```python
from build123d import *

# Parameters (mm, degrees)
SKETCH2_W                  = 60
SKETCH2_H                  = 60
BOSS_EXTRUDE1_DEPTH        = 7.5
BOSS_EXTRUDE2_DEPTH        = 15
FILLET1_R                  = 1
SKETCH4_R                  = 2.5
CUT_EXTRUDE1_DEPTH         = 57.024687639
CUT_EXTRUDE2_START         = -7.5
SKETCH5_R                  = 4.25
CUT_EXTRUDE2_DEPTH         = 7.5
CHAMFER3_SIZE              = 1
LPATTERN1_COUNT            = 5
LPATTERN1_PITCH            = 10
CHAMFER3_OF_LPATTERN1_SIZE = 1
CHAMFER1_SIZE              = 3
CHAMFER2_SIZE              = 1


# Read off the part's stored shape, not the designer's step: LPattern2
with BuildPart() as part:
    # Sketch2 → Boss-Extrude1 (new, symmetric)
    with BuildSketch(Plane(origin=(0, 0, 0), x_dir=(0, 1, 0), z_dir=(0, 0, 1))):
        Rectangle(SKETCH2_W, SKETCH2_H)
    extrude(amount=BOSS_EXTRUDE1_DEPTH, both=True)

    # Sketch3 → Boss-Extrude2 (add, through all)
    with BuildSketch(Plane.XY.offset(7.5)):
        Polygon((-15.943747687, 44.875), (-7.355662433, 30), (7.355662433, 30), (15.943747687, 44.875), align=None)
    extrude(amount=-BOSS_EXTRUDE2_DEPTH)

    # Fillet1
    fillet1_edges = [part.edges().sort_by_distance(p)[0] for p in [
        (-7.355662433, 30, 0),
        (-15.943747687, 44.875, 0),
        (15.943747687, 44.875, 0),
        (7.355662433, 30, 0),
    ]]
    fillet(fillet1_edges, radius=FILLET1_R)

    # Sketch4 → Cut-Extrude1 (cut, symmetric)
    with BuildSketch(Plane.XY.offset(7.5)):
        with Locations((20, -20)):
            Circle(SKETCH4_R)
    cut_extrude1 = extrude(amount=CUT_EXTRUDE1_DEPTH, both=True, mode=Mode.SUBTRACT)

    # Sketch5 → Cut-Extrude2 (cut)
    with BuildSketch(Plane.XY.offset(7.5).offset(CUT_EXTRUDE2_START)):
        with Locations((20, -20)):
            Circle(SKETCH5_R)
    cut_extrude2 = extrude(amount=CUT_EXTRUDE2_DEPTH, mode=Mode.SUBTRACT)

    # Chamfer3
    chamfer3_edges = [part.edges().sort_by_distance(p)[0] for p in [
        (15.75, -20, 0),
    ]]
    chamfer(chamfer3_edges, length=CHAMFER3_SIZE)

    # LPattern1: Cut-Extrude1, Cut-Extrude2 ×5
    with Locations(*[(-i * LPATTERN1_PITCH, 0, 0) for i in range(1, LPATTERN1_COUNT)]):
        add(cut_extrude1, mode=Mode.SUBTRACT)
        add(cut_extrude2, mode=Mode.SUBTRACT)

    # Chamfer3 of LPattern1
    chamfer3_of_lpattern1_edges = [part.edges().sort_by_distance(p)[0] for p in [
        (5.75, -20, 0),
        (-4.25, -20, 0),
        (-14.25, -20, 0),
        (-24.25, -20, 0),
    ]]
    chamfer(chamfer3_of_lpattern1_edges, length=CHAMFER3_OF_LPATTERN1_SIZE)

    # LPattern2 outline → LPattern2 (revolve, cut)
    with BuildSketch(Plane(origin=(-20, 20, 0), x_dir=(1, 0, 0), z_dir=(0, -1, 0))):
        Polygon((0, -7.5), (2.5, -7.5), (2.5, 0), (3.25, 0), (4.25, 1), (4.25, 7.5), (0, 7.5), align=None)
    revolve(axis=Axis((-20, 20, 0), (0, 0, 1)), mode=Mode.SUBTRACT)

    # LPattern2 2 outline → LPattern2 2 (revolve, cut)
    with BuildSketch(Plane(origin=(-10, 20, 0), x_dir=(1, 0, 0), z_dir=(0, -1, 0))):
        Polygon((0, -7.5), (2.5, -7.5), (2.5, 0), (3.25, 0), (4.25, 1), (4.25, 7.5), (0, 7.5), align=None)
    revolve(axis=Axis((-10, 20, 0), (0, 0, 1)), mode=Mode.SUBTRACT)

    # LPattern2 3 outline → LPattern2 3 (revolve, cut)
    with BuildSketch(Plane.XZ.offset(-20)):
        Polygon((0, -7.5), (2.5, -7.5), (2.5, 0), (3.25, 0), (4.25, 1), (4.25, 7.5), (0, 7.5), align=None)
    revolve(axis=Axis((0, 20, 0), (0, 0, 1)), mode=Mode.SUBTRACT)

    # LPattern2 4 outline → LPattern2 4 (revolve, cut)
    with BuildSketch(Plane(origin=(10, 20, 0), x_dir=(1, 0, 0), z_dir=(0, -1, 0))):
        Polygon((0, -7.5), (2.5, -7.5), (2.5, 0), (3.25, 0), (4.25, 1), (4.25, 7.5), (0, 7.5), align=None)
    revolve(axis=Axis((10, 20, 0), (0, 0, 1)), mode=Mode.SUBTRACT)

    # LPattern2 5 outline → LPattern2 5 (revolve, cut)
    with BuildSketch(Plane(origin=(20, 20, 0), x_dir=(1, 0, 0), z_dir=(0, -1, 0))):
        Polygon((0, -7.5), (2.5, -7.5), (2.5, 0), (3.25, 0), (4.25, 1), (4.25, 7.5), (0, 7.5), align=None)
    revolve(axis=Axis((20, 20, 0), (0, 0, 1)), mode=Mode.SUBTRACT)

    # LPattern2 6 outline → LPattern2 6 (revolve, cut)
    with BuildSketch(Plane(origin=(-20, 0, 0), x_dir=(1, 0, 0), z_dir=(0, -1, 0))):
        Polygon((0, -7.5), (2.5, -7.5), (2.5, 0), (3.25, 0), (4.25, 1), (4.25, 7.5), (0, 7.5), align=None)
    revolve(axis=Axis((-20, 0, 0), (0, 0, 1)), mode=Mode.SUBTRACT)

    # LPattern2 7 outline → LPattern2 7 (revolve, cut)
    with BuildSketch(Plane(origin=(-10, 0, 0), x_dir=(1, 0, 0), z_dir=(0, -1, 0))):
        Polygon((0, -7.5), (2.5, -7.5), (2.5, 0), (3.25, 0), (4.25, 1), (4.25, 7.5), (0, 7.5), align=None)
    revolve(axis=Axis((-10, 0, 0), (0, 0, 1)), mode=Mode.SUBTRACT)

    # LPattern2 8 outline → LPattern2 8 (revolve, cut)
    with BuildSketch(Plane.XZ):
        Polygon((0, -7.5), (2.5, -7.5), (2.5, 0), (3.25, 0), (4.25, 1), (4.25, 7.5), (0, 7.5), align=None)
    revolve(axis=Axis((0, 0, 0), (0, 0, 1)), mode=Mode.SUBTRACT)

    # LPattern2 9 outline → LPattern2 9 (revolve, cut)
    with BuildSketch(Plane(origin=(10, 0, 0), x_dir=(1, 0, 0), z_dir=(0, -1, 0))):
        Polygon((0, -7.5), (2.5, -7.5), (2.5, 0), (3.25, 0), (4.25, 1), (4.25, 7.5), (0, 7.5), align=None)
    revolve(axis=Axis((10, 0, 0), (0, 0, 1)), mode=Mode.SUBTRACT)

    # LPattern2 10 outline → LPattern2 10 (revolve, cut)
    with BuildSketch(Plane(origin=(20, 0, 0), x_dir=(1, 0, 0), z_dir=(0, -1, 0))):
        Polygon((0, -7.5), (2.5, -7.5), (2.5, 0), (3.25, 0), (4.25, 1), (4.25, 7.5), (0, 7.5), align=None)
    revolve(axis=Axis((20, 0, 0), (0, 0, 1)), mode=Mode.SUBTRACT)

    # Chamfer1
    chamfer1_edges = [part.edges().sort_by_distance(p)[0] for p in [
        (-30, -30, 0),
        (-30, 30, 0),
        (30, 30, 0),
        (30, -30, 0),
    ]]
    chamfer(chamfer1_edges, length=CHAMFER1_SIZE)

    # Chamfer2
    chamfer2_edges = [part.edges().sort_by_distance(p)[0] for p in [
        (11.64970506, 37.4375, 7.5),
        (-30, 0, -7.5),
        (-30, 0, 7.5),
        (11.64970506, 37.4375, -7.5),
        (30, 0, -7.5),
        (0, -30, -7.5),
        (-18.04385662, 30, -7.5),
        (28.5, 28.5, -7.5),
        (28.5, -28.5, -7.5),
        (-28.5, -28.5, -7.5),
        (-28.5, 28.5, -7.5),
        (-18.04385662, 30, 7.5),
        (0, -30, 7.5),
        (30, 0, 7.5),
        (28.5, 28.5, 7.5),
        (28.5, -28.5, 7.5),
        (-28.5, -28.5, 7.5),
        (-28.5, 28.5, 7.5),
        (18.04385662, 30, 7.5),
        (0, 44.875, 7.5),
        (-11.64970506, 37.4375, 7.5),
        (-15.077722283, 44.375, 7.5),
        (15.077722283, 44.375, 7.5),
        (0, 44.875, -7.5),
        (-11.64970506, 37.4375, -7.5),
        (18.04385662, 30, -7.5),
        (-15.077722283, 44.375, -7.5),
        (15.077722283, 44.375, -7.5),
        (-8.221687836, 30.5, 7.5),
        (-8.221687836, 30.5, -7.5),
        (8.221687836, 30.5, 7.5),
        (8.221687836, 30.5, -7.5),
    ]]
    chamfer(chamfer2_edges, length=CHAMFER2_SIZE - 0.0001)  # a hair under: the kernel refuses the full size


solid = part.part
```
Part model, mm, in its own coordinate system. A direction names the side the tool comes from. Round coordinates to 2 decimals unless told otherwise and drop trailing zeros. Put each result on its own line as item: value. Start each with the question number.
1. Drop flat-ended pins along their axis: pin 1 (4.5 mm diameter, centred on x = 20, y = 0, fed in from -Z); pin 2 (2 mm diameter, centred on x = 18.5, y = -19.5, fed in from +Z); pin 3 (8 mm diameter, centred on x = 20, y = 20, fed in from +Z); pin 4 (2 mm diameter, centred on x = -20, z = -3, fed in from +Y). Give the stop position or say it passes through.
2. Two-plate mould, pull along Y, no slides. Class faces 1 (the face through (30, 0, 0)), 2 (the face through (-11.259, 37.774, -7.007)), 3 (the face through (-28.13, -28.172, 6.993)): +Y half, -Y half, draft (parallel to the pull), parting line (faces both ways), or undercut.
3. Drill centre lines: probe 1 along Y at (x, z) = (-20, -2.75); probe 2 along Y at (x, z) = (10, 4.25) (3 decimals); probe 3 along X at (y, z) = (1, -2.25). Where is each one in solid material? Low to high. Write a range as [from, to].
4. Slice it at A-A on z = 5. State how many separate pieces and enclosed holes the cut face has, then the cut area to 3 significant figures.
5. Tool access for faces 4 (the face through (18, 30, 0)), 5 (the face through (11.16, 37.61, -7.01)), 6 (the face through (2.285, 3.584, 4.296)), 7 (the face through (17.5, -19.9, -3.7)): list every direction of +Z, -Z, +X, -X, +Y, -Y with a clear straight run to the whole face (end or side of a thin tool).
Findings:
1. pin 1: through
1. pin 2: z = 0
1. pin 3: z = 0.75
1. pin 4: y = 30
2. face 1: draft
2. face 2: undercut
2. face 3: -Y half
3. probe 1: [-30, -22.5], [-17.5, -2.5], [2.5, 17.5], [22.5, 30]
3. probe 2: [-30, -24.25], [-15.75, -4.25], [4.25, 15.75], [24.25, 30], [34.58, 44.875]
3. probe 3: [-30, -22.29], [-17.71, -12.29], [-7.71, -2.29], [2.29, 7.71], [12.29, 17.71], [22.29, 30]
4. separate pieces: 1
4. enclosed holes: 15
4. area: 3,080 mm2
5. face 4: +Z, -Z, +X
5. face 5: -Z, +X
5. face 6: +Z
5. face 7: +Z, -Z
